Could you check a few things on this drawing? It's one solid part, dimensions in mm from its lowest x, y, z. A direction names the side the tool comes from. Round coordinates to 2 decimals unless told otherwise and drop trailing zeros. Loops run counter-clockwise (first coordinate to the right, second up) from the corner with the lowest first, then second, coordinate; pieces in that order, holes last. Notation, with made-up numbers: M 52,-18.5 L 62,-18.5 A26 cw 62,7.5 Z; hole C 35,42.5 d1. An arc over 180 degrees is marked long. Write each question's results on one line, items separated by ' | '. Start each with the question number.
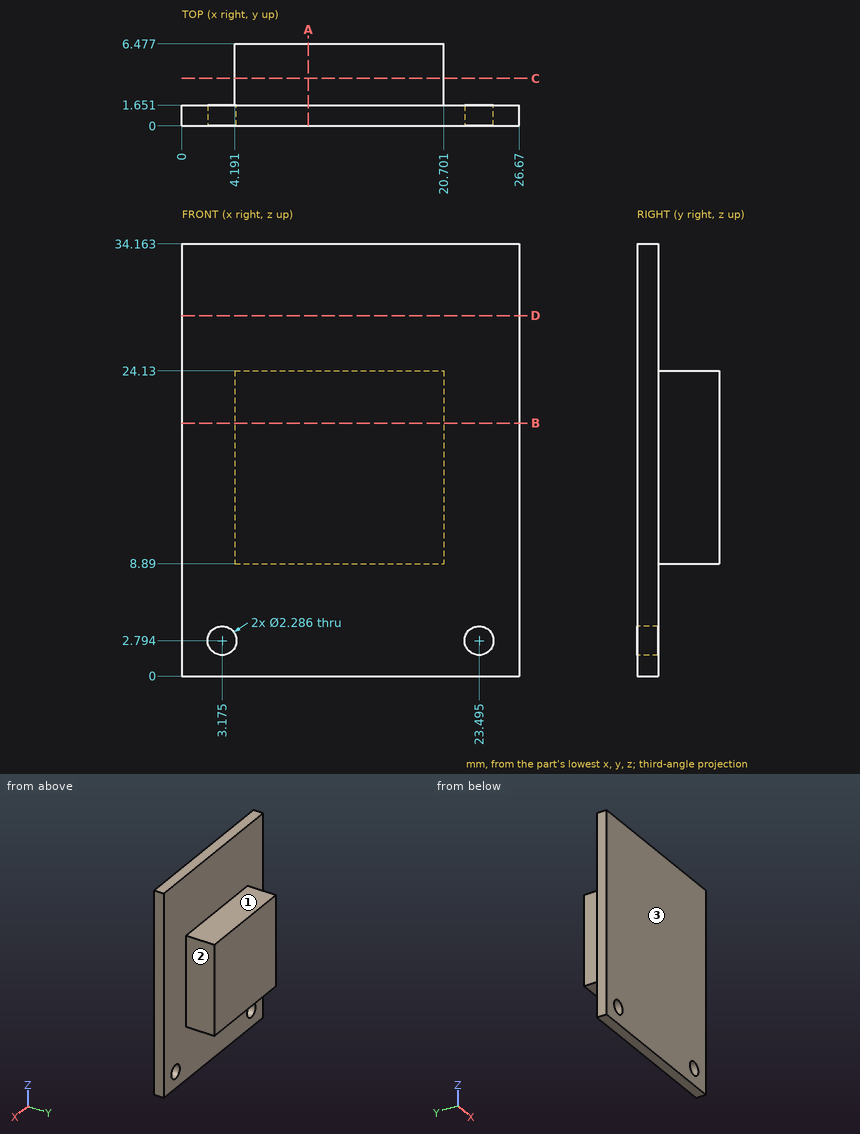
1. For pin 1 (1 mm diameter, centred on x = 20.5, y = 5.5, fed in from -Z); pin 2 (1.4 mm diameter, centred on y = 4, z = 20, fed in from -X); pin 3 (2.5 mm diameter, centred on x = 23.495, z = 2.794, fed in from +Y), each with a flat end and sliding along its axis, tell me the tip position at first contact or that it passes through.
2. I need wall thicknesses on line 1 along X through (y, z) = (0.75, 3); line 2 along Z through (x, y) = (8.5, 5.75); line 3 along Y through (x, z) = (21.5, 22). Which ranges of each line are inside material? Lowest first, please.
3. I want a section at D-D on z = 28.5. List the corners of the cut face in (x, y) for me, plus the area to 3 significant figures.
4. I want a section at C-C on y = 3.75. List the corners of the cut face in (x, z) for me.
5. Which directions (+Z, -Z, +X, -X, +Y, -Y) give clear straight access to the entire face, cutting with the end or side of a thin tool? Please do the marked faces 1, 2 and 3.
6. I want a section at A-A on x = 10. List the corners of the cut face in (y, z) for me.
7. I want a section at B-B on z = 20. List the corners of the cut face in (x, y) for me, plus the area to 3 significant figures.
Outcome:
1) pin 1: z = 8.89 | pin 2: x = 4.19 | pin 3: y = 1.65
2) line 1: 0 to 2.05, 4.3 to 22.37, 24.62 to 26.67 | line 2: 8.89 to 24.13 | line 3: 0 to 1.65
3) outline: M 0,0 L 26.67,0 L 26.67,1.65 L 0,1.65 Z | area: 44.0 mm2
4) outline: M 4.19,8.89 L 20.7,8.89 L 20.7,24.13 L 4.19,24.13 Z
5) face 1: +Z, +X, -X, +Y | face 2: +Z, -Z, +X, +Y | face 3: +Z, -Z, +X, -X, -Y
6) outline: M 0,0 L 1.65,0 L 1.65,8.89 L 6.48,8.89 L 6.48,24.13 L 1.65,24.13 L 1.65,34.16 L 0,34.16 Z
7) outline: M 0,0 L 26.67,0 L 26.67,1.65 L 20.7,1.65 L 20.7,6.48 L 4.19,6.48 L 4.19,1.65 L 0,1.65 Z | area: 124 mm2
